from build123d import *

# Parameters (mm, degrees)
SKETCH1_R           = 1.75
BOSS_EXTRUDE1_DEPTH = 3.5
THREAD1_PITCH       = 0.5


with BuildPart() as part:
    # Sketch1 → Boss-Extrude1 (new body)
    with BuildSketch(Plane.XY):
        Polygon((3.954849344, 0), (1.977424672, 3.425), (-1.977424672, 3.425), (-3.954849344, 0), (-1.977424672, -3.425), (1.977424672, -3.425), align=None)
        Circle(SKETCH1_R, mode=Mode.SUBTRACT)
    extrude(amount=BOSS_EXTRUDE1_DEPTH)

    # Thread1: the profile of Thread Profile1 profile screwed along a right-hand helix of 2 turns, 6 arcs to a turn; built about Z, then put on its axis
    thread1_z = Axis((0, 0, 0), (0, 0, 1))
    thread1_corners = [(1.7503, 0, -0.000173205), (1.7503, 0, 0.437673204), (1.479367063, 0, 0.281249999), (1.479367062, 0, 0.156249999)]
    with BuildLine(mode=Mode.PRIVATE) as thread1_profile:
        Line(thread1_corners[0], thread1_corners[1])
        Line(thread1_corners[1], thread1_corners[2])
        Line(thread1_corners[2], thread1_corners[3])
        Line(thread1_corners[3], thread1_corners[0])
    thread1_cap = Face(thread1_profile.wire())
    thread1_turn_angles = [0, 30, 60, 90, 120, 150, 180, 210, 240, 270, 300, 330, 360]
    thread1_turn_weights = [1, 0.8660254037844387, 1, 0.8660254037844387, 1, 0.8660254037844387, 1, 0.8660254037844387, 1, 0.8660254037844387, 1, 0.8660254037844387, 1]
    thread1_turn_rails = [Edge.make_bspline([Vector(p[0], p[1], 0).rotate(thread1_z, thread1_turn_angles[k]) / thread1_turn_weights[k] + Vector(0, 0, p[2] + THREAD1_PITCH * thread1_turn_angles[k] / 360) for k in range(13)], [0, 0, 0, 1, 1, 2, 2, 3, 3, 4, 4, 5, 5, 6, 6, 6], 2, thread1_turn_weights) for p in thread1_corners]
    thread1_turn_sides = [Face.make_surface_from_curves(thread1_turn_rails[p[0]], thread1_turn_rails[p[1]]) for p in [(0, 1), (1, 2), (2, 3), (3, 0)]]
    thread1 = Plane(origin=(0, 0, 3.5), x_dir=(-1, 0, 0), z_dir=(0, 0, -1)) * Solid(Shell([*[p.moved(Location((0, 0, THREAD1_PITCH * i))) for i in range(2) for p in thread1_turn_sides], thread1_cap, thread1_cap.rotate(thread1_z, 720).moved(Location((0, 0, THREAD1_PITCH * 720 / 360)))]))
    add(thread1)


solid = part.part
Part model, mm, in its own coordinate system. Round coordinates to 2 decimals unless told otherwise and drop trailing zeros. Loops run counter-clockwise (first coordinate to the right, second up) from the corner with the lowest first, then second, coordinate; pieces in that order, holes last. Notation, with made-up numbers: (-17.5, 81.25) - (7.5, 81.25) arc R31 cw to (7.5, 116.25) - close; hole circle Ø3 at (-31.5, 9). An arc over 180 degrees is marked (long way). Answer as a JSON object with one key per item and string values.
Item 1: Wall check: L1, parallel to Z at x = -1, y = 1.25; L2, parallel to X at y = 0.5, z = 0.45; L3, parallel to X at y = -0.75, z = 2.15. Give the ranges that are in metal, low to high.
Output:
{"L1": "2.58 to 2.84, 3.08 to 3.34", "L2": "-3.67 to -1.68, 1.68 to 3.67", "L3": "-3.52 to -1.48, 1.58 to 3.52"}
Item 2: Band-saw the part on C-C on x = -2.5. List the corners of the cut face in (y, z), plus the area to 3 significant figures.
Output:
{"outline": "(-2.52, 0) - (2.52, 0) - (2.52, 3.5) - (-2.52, 3.5) - close", "area": "17.6 mm2"}
Item 3: Band-saw the part on B-B on y = 2.75. List the corners of the cut face in (x, z), plus the area to 3 significant figures.
Output:
{"outline": "(-2.37, 0) - (2.37, 0) - (2.37, 3.5) - (-2.37, 3.5) - close", "area": "16.6 mm2"}
Item 4: Pin check, flat tip, straight feed: pin 1 (2 mm diameter, centred on x = 0, y = 0, fed in from +Z). Stop position of the tip, or through.
Output:
{"pin 1": "through"}
Item 5: Band-saw the part on A-A on z = 1.6. List the corners of the cut face in (x, y) (3 decimals).
Output:
{"outline": "(-3.955, 0) - (-1.977, -3.425) - (1.977, -3.425) - (3.955, 0) - (1.977, 3.425) - (-1.977, 3.425) - close; hole circle Ø3.5 at (0, 0)"}
